Geometry: final body of the model. Coordinates: model frame, mm. A direction names the side the tool comes from. Give positions to 0.01 mm unless a question says otherwise; leave off trailing zeros. Loops run counter-clockwise (first coordinate to the right, second up) from the corner with the lowest first, then second, coordinate; pieces in that order, holes last. Notation, with made-up numbers: (-8, 28) - (14, 28) arc R20 ccw to (14, 40) - close; hole circle Ø2 at (26.5, 1.25). An arc over 180 degrees is marked (long way). Answer in a Markdown table with one row per item.
from build123d import *

# Parameters (mm, degrees)
F0_W       = 450
F0_H       = 190
F1_DEPTH   = 25
F2_SIZE    = 10
F3_R       = 35
F3_R_2     = 17.5
F4_DEPTH   = 3
F5_SIZE2   = 1.8198511713
F5_SIZE    = 5
F5_2_SIZE2 = 1.8198511713
F5_2_SIZE  = 5
F5_3_SIZE2 = 1.8198511713
F5_3_SIZE  = 5
F5_4_SIZE2 = 1.8198511713
F5_4_SIZE  = 5
F5_5_SIZE2 = 1.8198511713
F5_5_SIZE  = 5
F5_6_SIZE2 = 1.8198511713
F5_6_SIZE  = 5
F5_7_SIZE2 = 1.8198511713
F5_7_SIZE  = 5
F5_8_SIZE2 = 1.8198511713
F5_8_SIZE  = 5
F6_R       = 10
F7_DEPTH   = 65


with BuildPart() as f1:
    # F0 (on Top) → F1 (new body)
    with BuildSketch(Plane.XY):
        with Locations((-7.6082125306, 13.8156425953)):
            Rectangle(F0_W, F0_H)
    extrude(amount=F1_DEPTH)

    # F2
    f2_edges = [f1.edges().sort_by_distance(p)[0] for p in [
        (-232.608213, 13.815643, 25),
        (217.391787, 13.815643, 25),
        (-7.608213, -81.184357, 25),
    ]]
    chamfer(f2_edges, length=F2_SIZE)

    # F3 (on face) → F4 (join)
    with BuildSketch(Plane.XY.offset(25)):
        with Locations((-152.3020284353, 18.9153849379)):
            Circle(F3_R)
        with Locations((-42.2719009221, 28.5504534841)):
            Circle(F3_R_2)
        with Locations((-42.2719009221, -17.1180190518)):
            Circle(F3_R_2)
        with Locations((7.2203539312, 43.2646488771)):
            Circle(F3_R_2)
        with Locations((7.2203539312, -2.4038236588)):
            Circle(F3_R_2)
        with Locations((53.6563685164, 21.6214338434)):
            Circle(F3_R_2)
        with Locations((170.8431290463, 80.1688283682)):
            Circle(F3_R_2)
        with Locations((125.1746565104, 80.1688283682)):
            Circle(F3_R_2)
        with Locations((53.6563685164, -24.0470386925)):
            Circle(F3_R_2)
    extrude(amount=F4_DEPTH)

    # F5
    f5_edges = [f1.edges().sort_by_distance(p)[0] for p in [
        (-59.771901, -17.118019, 28),
    ]]
    f5_side = f1.faces().sort_by_distance((-42.271901, -17.118019, 28))[0]
    chamfer(f5_edges, length=F5_SIZE, length2=F5_SIZE2, reference=f5_side)

    # F5#2
    f5_2_edges = [f1.edges().sort_by_distance(p)[0] for p in [
        (36.156369, -24.047039, 28),
    ]]
    f5_2_side = f1.faces().sort_by_distance((53.656369, -24.047039, 28))[0]
    chamfer(f5_2_edges, length=F5_2_SIZE, length2=F5_2_SIZE2, reference=f5_2_side)

    # F5#3
    f5_3_edges = [f1.edges().sort_by_distance(p)[0] for p in [
        (-10.279646, -2.403824, 28),
    ]]
    f5_3_side = f1.faces().sort_by_distance((7.220354, -2.403824, 28))[0]
    chamfer(f5_3_edges, length=F5_3_SIZE, length2=F5_3_SIZE2, reference=f5_3_side)

    # F5#4
    f5_4_edges = [f1.edges().sort_by_distance(p)[0] for p in [
        (36.156369, 21.621434, 28),
    ]]
    f5_4_side = f1.faces().sort_by_distance((53.656369, 21.621434, 28))[0]
    chamfer(f5_4_edges, length=F5_4_SIZE, length2=F5_4_SIZE2, reference=f5_4_side)

    # F5#5
    f5_5_edges = [f1.edges().sort_by_distance(p)[0] for p in [
        (-59.771901, 28.550453, 28),
    ]]
    f5_5_side = f1.faces().sort_by_distance((-42.271901, 28.550453, 28))[0]
    chamfer(f5_5_edges, length=F5_5_SIZE, length2=F5_5_SIZE2, reference=f5_5_side)

    # F5#6
    f5_6_edges = [f1.edges().sort_by_distance(p)[0] for p in [
        (-10.279646, 43.264649, 28),
    ]]
    f5_6_side = f1.faces().sort_by_distance((7.220354, 43.264649, 28))[0]
    chamfer(f5_6_edges, length=F5_6_SIZE, length2=F5_6_SIZE2, reference=f5_6_side)

    # F5#7
    f5_7_edges = [f1.edges().sort_by_distance(p)[0] for p in [
        (107.674657, 80.168828, 28),
    ]]
    f5_7_side = f1.faces().sort_by_distance((125.174657, 80.168828, 28))[0]
    chamfer(f5_7_edges, length=F5_7_SIZE, length2=F5_7_SIZE2, reference=f5_7_side)

    # F5#8
    f5_8_edges = [f1.edges().sort_by_distance(p)[0] for p in [
        (153.343129, 80.168828, 28),
    ]]
    f5_8_side = f1.faces().sort_by_distance((170.843129, 80.168828, 28))[0]
    chamfer(f5_8_edges, length=F5_8_SIZE, length2=F5_8_SIZE2, reference=f5_8_side)

    # F6 (on face) → F7 (join)
    with BuildSketch(Plane.XY.offset(28)):
        with Locations((-151.709437467, 19.1692207788)):
            Circle(F6_R)
    extrude(amount=F7_DEPTH)


solid = f1.part
Q1. Cut plane D-D (z = 73). Output: boundary loops of the cut face in (x, y).
Check values:
| item | result |
|---|---|
| outline | circle Ø20 at (-151.71, 19.17) |
Q2. First-contact query: pin 1 (8 mm diameter, centred on y = 67.5, z = 26.5, fed in from -X); pin 2 (12.5 mm diameter, centred on x = 175, y = 79, fed in from +Z); pin 3 (12 mm diameter, centred on x = 44, y = 4, fed in from +Z); pin 4 (1.5 mm diameter, centred on x = -115, z = 15.5, fed in from -Y). Flat tips, straight axial feed; report the tip coordinate or a pass-through.
Check values:
| item | result |
|---|---|
| pin 1 | x = -225.11 |
| pin 2 | z = 28 |
| pin 3 | z = 27.42 |
| pin 4 | y = -81.18 |
Q3. Cut plane B-B (x = 147). Output: boundary loops of the cut face in (y, z), and give its area (3 significant figures).
Check values:
| item | result |
|---|---|
| outline | (-81.18, 0) - (108.82, 0) - (108.82, 25) - (-71.18, 25) - (-81.18, 15) - close |
| area | 4,700 mm² |
Q4. Draft query along Y for faces 4 (the flat face through (-11, -81.184, 7)), 5 (the cylindrical face through (-5.7, 9.4, 25.6)), 6 (the cylindrical face through (-159.889, -15.252, 26.479)), 7 (the flat face through (7, 43, 28)). Return one class per face: pulls with the +Y half, pulls with the -Y half, needs draft (parallel to the pull), parting line crosses it, or undercut.
Check values:
| item | result |
|---|---|
| face 4 | pulls with the -Y half |
| face 5 | undercut |
| face 6 | parting line crosses it |
| face 7 | needs draft |
Q5. Cut plane A-A (y = -51.5). Output: boundary loops of the cut face in (x, z).
Check values:
| item | result |
|---|---|
| outline | (-232.61, 0) - (217.39, 0) - (217.39, 15) - (207.39, 25) - (-222.61, 25) - (-232.61, 15) - close |
Q6. Material intervals for line 1 along Z through (x, y) = (-53, 71); line 2 along Z through (x, y) = (126.5, 89.5); line 3 along Y through (x, z) = (-61, 21), sorted ascending.
Check values:
| item | result |
|---|---|
| line 1 | 0 to 25 |
| line 2 | 0 to 28 |
| line 3 | -75.18 to 108.82 |
Q7. Cut plane C-C (x = -174). Output: boundary loops of the cut face in (y, z).
Check values:
| item | result |
|---|---|
| outline | (-81.18, 0) - (108.82, 0) - (108.82, 25) - (46.38, 25) - (46.38, 28) - (-8.55, 28) - (-8.55, 25) - (-71.18, 25) - (-81.18, 15) - close |
Q8. Reachability of faces 1 (the flat face through (-42, -17, 28)), 2 (the flat face through (53, 22, 28)), 3 (the flat face through (-11, 20, 25)) from +Z, -Z, +X, -X, +Y, -Y: full face, straight path, thin tool, end or side. Return the list, or none.
Check values:
| item | result |
|---|---|
| face 1 | +Z, +X, -X, +Y, -Y |
| face 2 | +Z, +X, +Y, -Y |
| face 3 | +Z |
